from build123d import *

# Parameters (mm, degrees)
BOSS_EXTRUDE1_DEPTH = 5
FILLET1_R           = 1
FILLET3_R           = 0.5


with BuildPart() as part:
    # Sketch1 → Boss-Extrude1 (new body)
    with BuildSketch(Plane.XY):
        with BuildLine():
            Line((-6.367771102, 10.5), (-7.053492803, 0.482844987))
            ThreePointArc((-7.053492803, 0.482844987), (-6.379046634, -3.048387121), (-4.055185405, -5.791404953))
            Line((-4.055185405, -5.791404953), (-2.908032532, -4.153100865))
            ThreePointArc((-2.908032532, -4.153100865), (-5.058941361, 0.334682398), (-2.335572735, 4.5))
            Line((-2.335572735, 4.5), (-4.5, 4.5))
            Line((-4.5, 4.5), (-4.5, 8.5))
            Line((-4.5, 8.5), (4.5, 8.5))
            Line((4.5, 8.5), (4.5, 4.5))
            Line((4.5, 4.5), (2.335572735, 4.5))
            ThreePointArc((2.335572735, 4.5), (4.332796658, 2.63282607), (5.07, 0))
            ThreePointArc((5.07, 0), (4.497144924, -2.341065469), (2.908032532, -4.153100865))
            Line((2.908032532, -4.153100865), (4.055185405, -5.791404953))
            ThreePointArc((4.055185405, -5.791404953), (6.379046634, -3.048387121), (7.053492803, 0.482844987))
            Line((7.053492803, 0.482844987), (6.367771102, 10.5))
            Line((6.367771102, 10.5), (-6.367771102, 10.5))
        make_face()
    extrude(amount=BOSS_EXTRUDE1_DEPTH)

    # Fillet1
    fillet1_edges = [part.edges().sort_by_distance(p)[0] for p in [
        (4.055185405, -5.791404953, 2.5),
        (2.908032532, -4.153100865, 2.5),
        (-4.055185405, -5.791404953, 2.5),
        (-2.908032532, -4.153100865, 2.5),
    ]]
    fillet(fillet1_edges, radius=FILLET1_R - 0.0001)  # a hair under: the kernel refuses the full size

    # Fillet3
    fillet3_edges = [part.edges().sort_by_distance(p)[0] for p in [
        (2.335572735, 4.5, 2.5),
        (-2.335572735, 4.5, 2.5),
    ]]
    fillet(fillet3_edges, radius=FILLET3_R)


solid = part.part
Read the model definition and answer for the solid it produces. Units are mm, in the model's axes. A direction names the side the tool comes from. Round coordinates to 2 decimals unless told otherwise and drop trailing zeros. Loops run counter-clockwise (first coordinate to the right, second up) from the corner with the lowest first, then second, coordinate; pieces in that order, holes last.
Q1. Section B-B on x = -4.25 is taken. Write down the section's boundary in (y, z).
Q2. Section A-A on y = 6.25 is taken. Write down the section's boundary in (x, z).
Q3. Section D-D on x = -2 is taken. Write down the section's boundary in (y, z).
Q4. Consider probe 1 along Y at (x, z) = (0.25, 0.85); probe 2 along X at (y, z) = (-1.25, 3.65); probe 3 along X at (y, z) = (0.5, 2.05). Determine where each line is inside the solid, lowest interval first.
Q5. Determine the mould class of faces 1 (the face through (-5, 4, 0)), 2 (the face through (-6.706, 5.562, 2.465)), 3 (the face through (-4.5, 6, 2)), 4 (the face through (4.5, 7, 2)) for opening direction Y: released by +Y, released by -Y, zero draft, split by the parting line, or undercut.
Q6. Each of these flat-tipped pins is pushed along its axis until it touches: pin 1 (1 mm diameter, centred on x = -0.5, y = 7.5, fed in from -Z); pin 2 (2 mm diameter, centred on x = 2, z = 3, fed in from -Y); pin 3 (2 mm diameter, centred on y = -3, z = 2, fed in from -X); pin 4 (3 mm diameter, centred on x = 2, z = 1.5, fed in from -Y). Where does it stop, or does it pass through?
Q7. Which of the six approach directions +Z, -Z, +X, -X, +Y, -Y give full straight-line access (tool end or side, diameter ignored) to faces 5 (the face through (-5, 4, 5)), 6 (the face through (-3.41, 4.18, 2.54))?
Output:
1. outline: (-5.33, 0) - (-2.76, 0) - (-2.76, 5) - (-5.33, 5) - close; (2.76, 0) - (4.5, 0) - (4.5, 5) - (2.76, 5) - close; (8.5, 0) - (10.5, 0) - (10.5, 5) - (8.5, 5) - close
2. outline: (-6.66, 0) - (-4.5, 0) - (-4.5, 5) - (-6.66, 5) - close; (4.5, 0) - (6.66, 0) - (6.66, 5) - (4.5, 5) - close
3. outline: (8.5, 0) - (10.5, 0) - (10.5, 5) - (8.5, 5) - close
4. probe 1: y = 8.5 to 10.5
4. probe 2: x = -6.96 to -4.91, 4.91 to 6.96
4. probe 3: x = -7.05 to -5.05, 5.05 to 7.05
5. face 1: zero draft
5. face 2: released by +Y
5. face 3: undercut
5. face 4: undercut
6. pin 1: passes through
6. pin 2: stops at y = 8.5
6. pin 3: stops at x = -6.78
6. pin 4: stops at y = -4.99
7. face 5: +Z, +X, -X, +Y, -Y
7. face 6: +Z, -Z
